Read the model definition and answer for the solid it produces. Units are mm, in the model's axes. A direction names the side the tool comes from. Give positions to 0.01 mm unless a question says otherwise; leave off trailing zeros. Loops run counter-clockwise (first coordinate to the right, second up) from the corner with the lowest first, then second, coordinate; pieces in that order, holes last. Notation, with made-up numbers: (29.25, 68.25) - (78.25, 68.25) arc R26 cw to (78.25, 104.25) - close; hole circle Ø11 at (20.25, 70). An arc over 180 degrees is marked (long way). Write each question's results on one line, items separated by ' | '. Start each with the question number.
Q1. Determine the mould class of faces 4 (the cylindrical face through (26.21, 1.14, 0.86)), 5 (the flat face through (2, 1, 26)), 6 (the flat face through (-17.948, 35, 13)) for opening direction Z: +Z half, -Z half, draft (parallel to the pull), parting line (faces both ways), or undercut.
Q2. Find the intervals of material crossed by line 1 (Y direction, x = 15, z = 16); line 2 (X direction, y = -8.5, z = 24.5); line 3 (X direction, y = 7.5, z = 24), in increasing order. Write a range as from..to.
Q3. The part is cut by section B-B, the plane z = 6.75. Write down the section's boundary in (x, y).
Q4. For faces 1 (the flat face through (-22.892, 0, 13)), 2 (the flat face through (2, 35, 20.888)), 3 (the flat face through (18, -20, 4)), determine the directions among +Z, -Z, +X, -X, +Y, -Y from which every point of the face is accessible in a straight line to the end or side of a thin tool.
Q5. The part is cut by section A-A, the plane x = -16.5. Write down the section's boundary in (y, z), plus the area to 3 significant figures.
Q6. Given pin 1 (0.9 mm diameter, centred on x = 18.5, y = -20, fed in from -Z); pin 2 (7.5 mm diameter, centred on x = 10.5, z = 15, fed in from +Y), each flat-ended and moving along its own axis, determine where each tip first touches the part or whether it passes through.
```python
from build123d import *

# Parameters (mm, degrees)
F0_W     = 50
F0_H     = 74
F1_DEPTH = 26
F2_W     = 40
F2_H     = 15
F3_DEPTH = 4.5
F5_R     = 3
F6_DEPTH = 4
F4_W     = 0.5
F4_H     = 2
F7_DEPTH = 0.2


with BuildPart() as f1:
    # F0 (on Top) → F1 (new body)
    with BuildSketch(Plane.XY):
        with Locations((2.1081687883, 0.6221723649)):
            Rectangle(F0_W, F0_H)
    extrude(amount=F1_DEPTH)

    # F2 (on face) → F3 (cut)
    with BuildSketch(Plane(origin=(0, 37.6221723649, 0), x_dir=(-1, 0, 0), z_dir=(0, 1, 0))):
        with Locations((-2.0523197204, 13.3878487907)):
            Rectangle(F2_W, F2_H)
    extrude(amount=-F3_DEPTH, mode=Mode.SUBTRACT)

    # F5
    f5_edges = [f1.edges().sort_by_distance(p)[0] for p in [
        (27.108169, 0.622172, 0),
        (27.108169, 0.622172, 26),
        (-22.891831, 0.622172, 0),
        (-22.891831, 0.622172, 26),
    ]]
    fillet(f5_edges, radius=F5_R)

    # F4 (on face) → F6 (cut)
    with BuildSketch(Plane(origin=(0, 0, 0), x_dir=(1, 0, 0), z_dir=(0, 0, -1))):
        with BuildLine():
            Line((18.1081687883, 20.3778276351), (18.1081687883, 18.8778276351))
            ThreePointArc((18.1081687883, 18.8778276351), (19.16882896, 19.3171674633), (19.6081687883, 20.3778276351))
            ThreePointArc((19.6081687883, 20.3778276351), (18.1081687883, 21.8778276351), (16.6081687883, 20.3778276351))
            Line((16.6081687883, 20.3778276351), (18.1081687883, 20.3778276351))
        make_face()
        with BuildLine():
            ThreePointArc((16.6081687883, 20.3778276351), (17.0475086165, 19.3171674633), (18.1081687883, 18.8778276351))
            Line((18.1081687883, 18.8778276351), (18.1081687883, 20.3778276351))
            Line((18.1081687883, 20.3778276351), (16.6081687883, 20.3778276351))
        make_face()
        with BuildLine():
            Line((-12.8918312117, 20.3778276351), (-11.3918312117, 20.3778276351))
            ThreePointArc((-11.3918312117, 20.3778276351), (-13.9524913835, 21.4384878068), (-12.8918312117, 18.8778276351))
            Line((-12.8918312117, 18.8778276351), (-12.8918312117, 20.3778276351))
        make_face()
        with BuildLine():
            ThreePointArc((-12.8918312117, 18.8778276351), (-11.83117104, 19.3171674633), (-11.3918312117, 20.3778276351))
            Line((-11.3918312117, 20.3778276351), (-12.8918312117, 20.3778276351))
            Line((-12.8918312117, 20.3778276351), (-12.8918312117, 18.8778276351))
        make_face()
        with BuildLine():
            ThreePointArc((18.1081687883, -8.1221723649), (16.6081687883, -9.6221723649), (18.1081687883, -11.1221723649))
            Line((18.1081687883, -11.1221723649), (18.1081687883, -9.6221723649))
            Line((18.1081687883, -9.6221723649), (18.1081687883, -8.1221723649))
        make_face()
        with BuildLine():
            Line((18.1081687883, -9.6221723649), (18.1081687883, -11.1221723649))
            ThreePointArc((18.1081687883, -11.1221723649), (19.16882896, -10.6828325367), (19.6081687883, -9.6221723649))
            ThreePointArc((19.6081687883, -9.6221723649), (19.16882896, -8.5615121932), (18.1081687883, -8.1221723649))
            Line((18.1081687883, -8.1221723649), (18.1081687883, -9.6221723649))
        make_face()
    extrude(amount=-F6_DEPTH, mode=Mode.SUBTRACT)

    # F4 (on face) → F7 (cut)
    with BuildSketch(Plane(origin=(0, 0, 0), x_dir=(1, 0, 0), z_dir=(0, 0, -1))):
        with Locations((-12.6418312117, 7.3778276351)):
            Rectangle(F4_W, F4_H)
    extrude(amount=-F7_DEPTH, mode=Mode.SUBTRACT)


solid = f1.part
```
Check sheet entries:
1) face 4: -Z half | face 5: +Z half | face 6: undercut
2) line 1: y = -36.38..33.12 | line 2: x = -22.49..26.71 | line 3: x = -22.72..26.94
3) outline: (-22.89, -36.38) - (27.11, -36.38) - (27.11, 37.62) - (22.05, 37.62) - (22.05, 33.12) - (-17.95, 33.12) - (-17.95, 37.62) - (-22.89, 37.62) - close
4) face 1: +Z, -Z, -X, +Y, -Y | face 2: +Y | face 3: -Z
5) outline: (-36.38, 0) - (37.62, 0) - (37.62, 5.89) - (33.12, 5.89) - (33.12, 20.89) - (37.62, 20.89) - (37.62, 26) - (-36.38, 26) - close | area: 1,860 mm^2
6) pin 1: stops at z = 4 | pin 2: stops at y = 33.12
